Verification items for the finished model (mm, model axes). Face numbers are marked on the shaded views. Give positions to 0.01 mm unless a question says otherwise; leave off trailing zeros. Loops run counter-clockwise (first coordinate to the right, second up) from the corner with the lowest first, then second, coordinate; pieces in that order, holes last. Notation, with made-up numbers: M 45.25,-9.75 L 93.25,-9.75 A21 cw 93.25,11.25 Z; hole C 51.25,-6 d7. An arc over 180 degrees is marked long. Use a Markdown table: item, result.
from build123d import *

# Parameters (mm, degrees)
SKETCH1_R           = 1.85
BOSS_EXTRUDE1_DEPTH = 3
SKETCH2_R           = 2.5
BOSS_EXTRUDE2_DEPTH = 0.2
DOME2_FACE_RADIUS   = 2.5
DOME2_HEIGHT        = 1.5


with BuildPart() as part:
    # Sketch1 → Boss-Extrude1 (new body)
    with BuildSketch(Plane(origin=(0, 0, 0), x_dir=(1, 0, 0), z_dir=(0, 1, 0))):
        with Locations(Location((0, 0, 0), (0, 0, 270))):
            Circle(SKETCH1_R)
    extrude(amount=BOSS_EXTRUDE1_DEPTH)

    # Sketch2 → Boss-Extrude2 (add)
    with BuildSketch(Plane(origin=(0, 3, 0), x_dir=(1, 0, 0), z_dir=(0, 1, 0))):
        with Locations(Location((0, 0, 0), (0, 0, 270))):
            Circle(SKETCH2_R)
    extrude(amount=BOSS_EXTRUDE2_DEPTH)

    # Dome2: a dome of height H over a round flat face of radius A is a cap of a sphere of radius (A * A + H * H) / (2 * H)
    dome2_r = (DOME2_FACE_RADIUS * DOME2_FACE_RADIUS + DOME2_HEIGHT * DOME2_HEIGHT) / (2 * DOME2_HEIGHT)
    dome2_base = Plane((0, 3.2, 0), z_dir=(0, 1, 0))
    with Locations(dome2_base.offset(DOME2_HEIGHT - dome2_r)):
        dome2_ball = Sphere(dome2_r, mode=Mode.PRIVATE)
    add(split(dome2_ball, bisect_by=dome2_base, keep=Keep.TOP, mode=Mode.PRIVATE))


solid = part.part
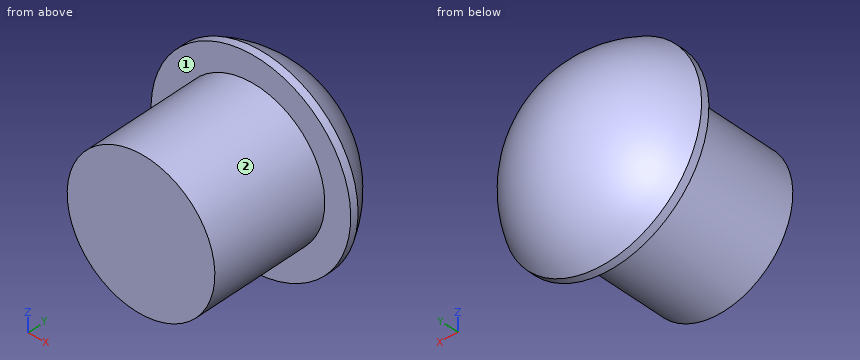
(1) Cross-section at A-A on z = 0. Record the cut outline in (x, y).
Results below:
| item | result |
|---|---|
| outline | M -2.5,3 L -1.85,3 L -1.85,0 L 1.85,0 L 1.85,3 L 2.5,3 L 2.5,3.2 A2.83 ccw -2.5,3.2 Z |
(2) Cross-section at D-D on z = 2. Record the cut outline in (x, y), then the cut area to 3 significant figures.
Results below:
| item | result |
|---|---|
| outline | M -1.5,3 L 1.5,3 L 1.5,3.2 A2.01 ccw -1.5,3.2 Z |
| area | 2.00 mm^2 |
(3) Gauge pin test, flat ends, axial feed: P1, Ø1, axis at y = 4, z = -1.5, coming from the -X side; P2, Ø2, axis at x = 1.5, y = 4, coming from the +Z side. Record the tip position at first contact, or that the pin passes through.
Results below:
| item | result |
|---|---|
| P1 | x = -1.89 |
| P2 | z = 2.33 |
(4) Draft check along Z on the marked faces 1 and 2. Enter one of: +Z half, -Z half, draft (parallel to the pull), parting line (faces both ways), or undercut.
Results below:
| item | result |
|---|---|
| face 1 | draft |
| face 2 | parting line |
(5) Cross-section at B-B on x = 0. Record the cut outline in (y, z), then the cut area to 3 significant figures.
Results below:
| item | result |
|---|---|
| outline | M 0,-1.85 L 3,-1.85 L 3,-2.5 L 3.2,-2.5 A2.83 ccw 3.2,2.5 L 3,2.5 L 3,1.85 L 0,1.85 Z |
| area | 17.4 mm^2 |
(6) Material ranges on line 1 (Z direction, x = 0.05, y = 2.25); line 2 (Y direction, x = -0.95, z = 1.1); line 3 (Y direction, x = 1.65, z = 0.9), recorded low to high.
Results below:
| item | result |
|---|---|
| line 1 | -1.85 to 1.85 |
| line 2 | 0 to 4.3 |
| line 3 | 3 to 3.99 |
(7) Cross-section at C-C on y = 2.9. Record the cut outline in (x, z), then the cut area to 3 significant figures.
Results below:
| item | result |
|---|---|
| outline | C 0,0 d3.7 |
| area | 10.8 mm^2 |
